from build123d import *

# Parameters (mm, degrees)
F1_DEPTH  = 22
F2_R      = 11.9
F3_DEPTH  = 1.75
F4_R      = 11.9
F5_DEPTH  = 1.75
F6_R      = 6.35
F6_R_2    = 4.75
F8_DEPTH  = 2
F7_R      = 6.35
F7_R_2    = 4.75
F9_DEPTH  = 2
F7_R_3    = 3
F10_DEPTH = 10
F6_R_3    = 3
F11_DEPTH = 10
F12_R     = 1.5
F13_R     = 0.8


with BuildPart() as f1:
    # F0 (on Top) → F1 (new body)
    with BuildSketch(Plane.XY):
        Polygon((6.680756, -12.7), (14.35, 0), (6.680756, 12.7), (-6.680756, 12.7), (-14.35, 0), (-6.680756, -12.7), align=None)
    extrude(amount=F1_DEPTH)

    # F2 (on face) → F3 (join)
    with BuildSketch(Plane.XY.offset(22)):
        Circle(F2_R)
    extrude(amount=F3_DEPTH)

    # F4 (on face) → F5 (join)
    with BuildSketch(Plane(origin=(0, 0, 0), x_dir=(1, 0, 0), z_dir=(0, 0, -1))):
        Circle(F4_R)
    extrude(amount=F5_DEPTH)

    # F6 (on face) → F8 (cut)
    with BuildSketch(Plane.XY.offset(23.75)):
        Circle(F6_R)
        Circle(F6_R_2, mode=Mode.SUBTRACT)
    extrude(amount=-F8_DEPTH, mode=Mode.SUBTRACT)

    # F7 (on face) → F9 (cut)
    with BuildSketch(Plane(origin=(0, 0, -1.75), x_dir=(1, 0, 0), z_dir=(0, 0, -1))):
        Circle(F7_R)
        Circle(F7_R_2, mode=Mode.SUBTRACT)
    extrude(amount=-F9_DEPTH, mode=Mode.SUBTRACT)

    # F7 (on face) → F10 (cut)
    with BuildSketch(Plane(origin=(0, 0, -1.75), x_dir=(1, 0, 0), z_dir=(0, 0, -1))):
        Circle(F7_R_3)
    extrude(amount=-F10_DEPTH, mode=Mode.SUBTRACT)

    # F6 (on face) → F11 (cut)
    with BuildSketch(Plane.XY.offset(23.75)):
        Circle(F6_R_3)
    extrude(amount=-F11_DEPTH, mode=Mode.SUBTRACT)

    # F12
    f12_edges = [f1.edges().sort_by_distance(p)[0] for p in [
        (-11.9, 0, 23.75),
        (-11.9, 0, -1.75),
    ]]
    fillet(f12_edges, radius=F12_R)

    # F13
    f13_edges = [f1.edges().sort_by_distance(p)[0] for p in [
        (-6.680756, 12.7, 11),
        (6.680756, 12.7, 11),
        (14.35, 0, 11),
        (6.680756, -12.7, 11),
        (-6.680756, -12.7, 11),
        (-14.35, 0, 11),
    ]]
    fillet(f13_edges, radius=F13_R)


solid = f1.part
Input: part model. Units: mm. Frame: model coordinates. A direction names the side the tool comes from. Give positions to 0.01 mm unless a question says otherwise; leave off trailing zeros. Write each loop counter-clockwise with the first axis right and the second up, starting at its lowest first coordinate (ties: lowest second). Pieces come first, ordered by that corner, then holes.
Q1. First-contact query: P1, Ø3, axis at x = 9.5, z = 18, coming from the -Y side; P2, Ø5, axis at x = 0, y = 0, coming from the -Z side; P3, Ø6.5, axis at x = 1.5, y = -1.5, coming from the -Z side; P4, Ø4, axis at x = -8.5, y = -9.5, coming from the +Z side. Flat tips, straight axial feed; report the tip coordinate or a pass-through.
Q2. Pull-direction query (Y, two-part tool) for faces 1 (the face through (-10.558, -6.28, 10.846)), 2 (the face through (2.192, 4.214, -0.764)), 3 (the face through (3, -1, 23.75)), 4 (the face through (14.215, -0.006, 11.154)); classes: pulls with the +Y half, pulls with the -Y half, needs draft (parallel to the pull), parting line crosses it, or undercut.
Q3. Set-up query: faces 5 (the face through (-1.38, 6.2, -0.76)), 6 (the face through (2.192, -4.214, 22.764)), 7 (the face through (-14.215, -0.006, 11.154)). Return all of +Z, -Z, +X, -X, +Y, -Y with unobstructed straight access to the full face (end or side cutting, diameter ignored); none if empty.
Q4. Section A-A, the plane z = 17. Output: boundary loops of the cut face in (x, y), plus the area to 3 significant figures.
Q5. Material intervals for probe 1 along X at (y, z) = (0, -0.25); probe 2 along Y at (x, z) = (0, -0.4); probe 3 along Y at (x, z) = (0, 4.75), sorted ascending.
Filled in:
1. P1: stops at y = -10.52
1. P2: stops at z = 8.25
1. P3: stops at z = -1.75
1. P4: stops at z = 23.71
2. face 1: pulls with the -Y half
2. face 2: undercut
2. face 3: needs draft
2. face 4: parting line crosses it
3. face 5: -Z
3. face 6: +Z
3. face 7: +Z, -Z, -X
4. outline: (-14.1, -0.41) - (-6.91, -12.31) arc R0.8 ccw to (-6.23, -12.7) - (6.23, -12.7) arc R0.8 ccw to (6.91, -12.31) - (14.1, -0.41) arc R0.8 ccw to (14.1, 0.41) - (6.91, 12.31) arc R0.8 ccw to (6.23, 12.7) - (-6.23, 12.7) arc R0.8 ccw to (-6.91, 12.31) - (-14.1, 0.41) arc R0.8 ccw to start; hole circle Ø6 at (0, 0)
4. area: 506 mm2
5. probe 1: x = -11.9 to -6.35, -4.75 to -3, 3 to 4.75, 6.35 to 11.9
5. probe 2: y = -11.89 to -6.35, -4.75 to -3, 3 to 4.75, 6.35 to 11.89
5. probe 3: y = -12.7 to -3, 3 to 12.7
